Input: dimensioned drawing with shaded views. Units: mm. Origin: part minimum x, y, z. A direction names the side the tool comes from. Coordinates: 2 decimals unless noted, no trailing zeros. Loops run counter-clockwise (first coordinate to the right, second up) from the corner with the lowest first, then second, coordinate; pieces in that order, holes last.
Item 1: Section D-D on y = 79. Return loops of the section in (x, z) (3 decimals), and give its area (3 significant figures).
Item 2: Ray query, line 1 along Z through (x, y) = (6.75, 22) (3 decimals); line 2 along X through (y, z) = (26, 26) (3 decimals); line 3 along X through (y, z) = (12, 14) (3 decimals). Return the intervals inside material, ascending.
Item 3: Contact query for flat-ended pins moving along their axis: P1, Ø6.5, axis at x = 9.5, y = 36, coming from the -Z side; P2, Ø1.5, axis at x = 2.5, z = 28.5, coming from the -Y side; P3, Ø6, axis at x = 9.5, z = 4, coming from the -Y side; P4, Ø6, axis at x = 10, z = 24.5, coming from the +Y side. Output: stop coordinate, or through.
Item 4: Pull-direction query (Z, two-part tool) for the marked faces 1, 2 and 3; classes: released by +Z, released by -Z, zero draft, split by the parting line, or undercut.
Item 5: Section C-C on y = 17. Return loops of the section in (x, z) (3 decimals), and give its area (3 significant figures).
Item 6: Section B-B on z = 5. Return loops of the section in (x, y) (3 decimals).
Item 7: Section A-A on x = 10.25. Return loops of the section in (y, z) (3 decimals), and give its area (3 significant figures).
Item 8: Reachability of the marked faces 4 and 5 from +Z, -Z, +X, -X, +Y, -Y: full face, straight path, thin tool, end or side. Return the list, or none.
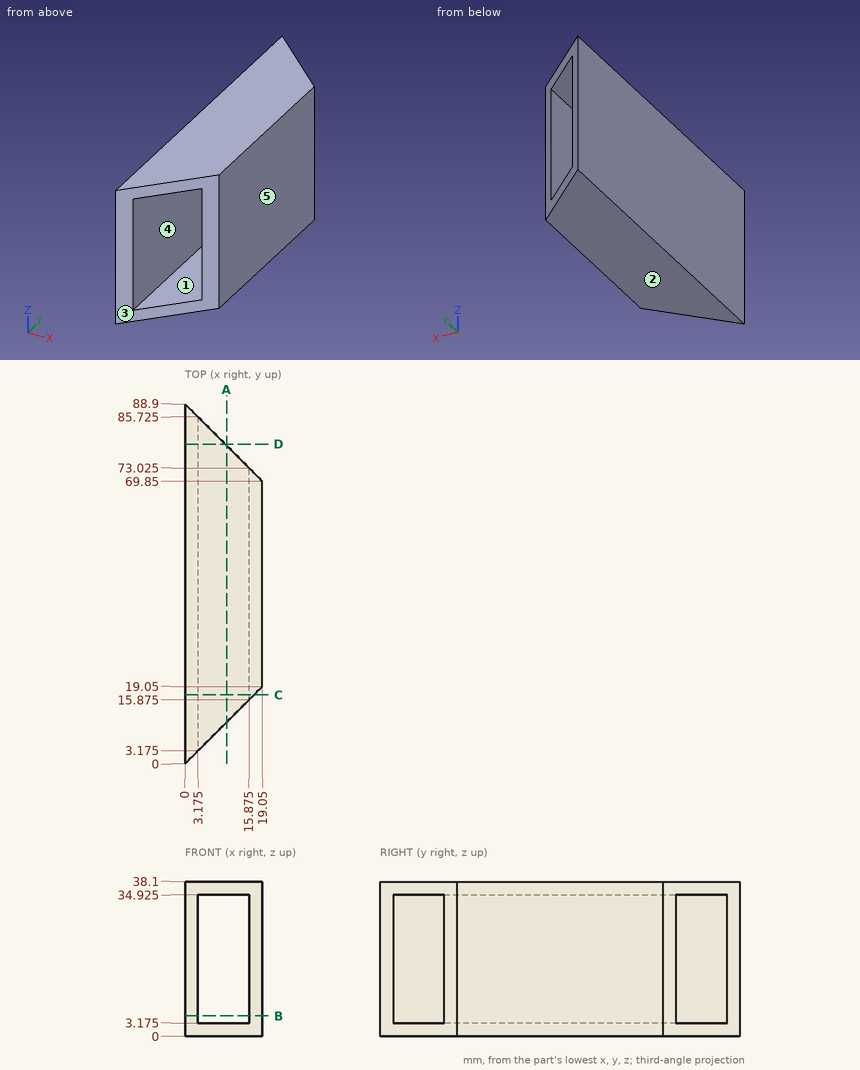
Results found:
1. outline: (0, 0) - (9.9, 0) - (9.9, 3.175) - (3.175, 3.175) - (3.175, 34.925) - (9.9, 34.925) - (9.9, 38.1) - (0, 38.1) - close
1. area: 164 mm2
2. line 1: z = 0 to 3.175, 34.925 to 38.1
2. line 2: x = 0 to 3.175, 15.875 to 19.05
2. line 3: x = 0 to 3.175
3. P1: stops at z = 0
3. P2: stops at y = 1.75
3. P3: stops at y = 6.62
3. P4: passes through
4. face 1: undercut
4. face 2: released by -Z
4. face 3: zero draft
5. outline: (0, 0) - (17, 0) - (17, 38.1) - (0, 38.1) - close; hole (3.175, 3.175) - (15.875, 3.175) - (15.875, 34.925) - (3.175, 34.925) - close
5. area: 244 mm2
6. outline: (0, 0) - (3.175, 3.175) - (3.175, 85.725) - (0, 88.9) - close; (15.875, 15.875) - (19.05, 19.05) - (19.05, 69.85) - (15.875, 73.025) - close
7. outline: (10.25, 0) - (78.65, 0) - (78.65, 3.175) - (10.25, 3.175) - close; (10.25, 34.925) - (78.65, 34.925) - (78.65, 38.1) - (10.25, 38.1) - close
7. area: 434 mm2
8. face 4: +Y, -Y
8. face 5: +Z, -Z, +X, +Y, -Y
